Design review of the part built by this model. Coordinates are the model's own, in mm. A direction names the side the tool comes from. Round coordinates to 2 decimals unless told otherwise and drop trailing zeros. Order: outer loops, then holes, each group sorted by start corner. A loop starts at its lowest first (then second) coordinate and runs counter-clockwise, first axis right, second up. Notation, with made-up numbers: (-22, 55) - (-18, 55) arc R21 cw to (-18, 67) - close; hole circle Ø6 at (-34.75, -6.75). An arc over 180 degrees is marked (long way). Answer as a JSON object with one key per item and string values. Group by question number.
from build123d import *

# Parameters (mm, degrees)
F0_R     = 7.625
F0_R_2   = 7
F1_DEPTH = 10.25
F2_DEPTH = 19.75
F3_DEPTH = 28.7
F4_SIZE  = 2.25


with BuildPart() as f1:
    # F0 (on Front) → F1 (new body)
    with BuildSketch(Plane.XZ):
        with BuildLine():
            Line((10.175, 10.075), (-10.075, 10.075))
            Line((-10.075, 10.075), (-10.075, 1.7320508076))
            ThreePointArc((-10.075, 1.7320508076), (-9.3429491924, 1), (-9.075, 0))
            ThreePointArc((-9.075, 0), (-9.3429491924, -1), (-10.075, -1.7320508076))
            Line((-10.075, -1.7320508076), (-10.075, -10.175))
            Line((-10.075, -10.175), (10.175, -10.175))
            Line((10.175, -10.175), (10.175, -1.7820508076))
            ThreePointArc((10.175, -1.7820508076), (9.175, -0.05), (10.175, 1.6820508076))
            Line((10.175, 1.6820508076), (10.175, 10.075))
        make_face()
        Circle(F0_R, mode=Mode.SUBTRACT)
        with BuildLine():
            Line((-10.075, -1.7320508076), (-10.075, 1.7320508076))
            ThreePointArc((-10.075, 1.7320508076), (-13.075, 0), (-10.075, -1.7320508076))
        make_face()
        with BuildLine():
            ThreePointArc((13.175, -0.05), (12.175, 1.6820508076), (10.175, 1.6820508076))
            Line((10.175, 1.6820508076), (10.175, -1.7820508076))
            ThreePointArc((10.175, -1.7820508076), (12.175, -1.7820508076), (13.175, -0.05))
        make_face()
        with BuildLine():
            Line((10.175, -1.7820508076), (10.175, 1.6820508076))
            ThreePointArc((10.175, 1.6820508076), (9.175, -0.05), (10.175, -1.7820508076))
        make_face()
        Circle(F0_R)
        Circle(F0_R_2, mode=Mode.SUBTRACT)
        Circle(F0_R_2)
        with BuildLine():
            ThreePointArc((-9.075, 0), (-9.3429491924, 1), (-10.075, 1.7320508076))
            Line((-10.075, 1.7320508076), (-10.075, -1.7320508076))
            ThreePointArc((-10.075, -1.7320508076), (-9.3429491924, -1), (-9.075, 0))
        make_face()
    extrude(amount=F1_DEPTH)

    # F0 (on Front) → F2 (join)
    with BuildSketch(Plane.XZ):
        Circle(F0_R)
        Circle(F0_R_2, mode=Mode.SUBTRACT)
        Circle(F0_R_2)
    extrude(amount=F2_DEPTH)

    # F0 (on Front) → F3 (join)
    with BuildSketch(Plane.XZ):
        Circle(F0_R_2)
    extrude(amount=F3_DEPTH)

    # F4
    f4_edges = [f1.edges().sort_by_distance(p)[0] for p in [
        (-10.075, -5.125, 10.075),
        (10.175, -5.125, 10.075),
        (10.175, -5.125, -10.175),
        (-10.075, -5.125, -10.175),
    ]]
    chamfer(f4_edges, length=F4_SIZE)


solid = f1.part
1. Take a section at B-B, the plane x = 0. Give the boundary of the cut face in (y, z) (3 decimals), then the cut area to 3 significant figures.
2. Take a section at D-D, the plane y = -18.5. Give the boundary of the cut face in (x, z) (3 decimals).
3. To check wall thickness, follow line 1 (Y direction, x = 7, z = 2.75); line 2 (Y direction, x = 8.25, z = 8.25); line 3 (X direction, y = -5.5, z = -3.25) (3 decimals). State the ranges of each line that lie inside material, in increasing order. Write a range as from..to.
4. Take a section at A-A, the plane y = -2.75. Give the boundary of the cut face in (x, z) (3 decimals).
5. Mouldability with a two-part tool opening along X and no side actions: class faces 3 (the cylindrical face through (-13.074, -5.053, 0.059)), 4 (the cylindrical face through (6.466, -24.162, -2.681)), 5 (the flat face through (-9, -5, -9)), 6 (the flat face through (7, -19.75, -2)) as pulls with the +X half, pulls with the -X half, needs draft (parallel to the pull), parting line crosses it, or undercut.
6. Clearance check with flat-ended pins moving along their axes: P1, Ø3, axis at y = -5.5, z = 4, coming from the -X side (3 decimals); P2, Ø3, axis at y = -4, z = 5, coming from the +X side (3 decimals); P3, Ø6, axis at x = -8.5, z = -6.5, coming from the -Y side. State where each tip first meets the part, or that it passes through.
7. Tool access review of faces 1 (the flat face through (9, -10.25, 0)), 2 (the flat face through (0, 0, 0)): name each direction out of +Z, -Z, +X, -X, +Y, -Y from which nothing blocks a thin tool from reaching the whole face with its end or side.
8. Take a section at C-C, the plane z = -5.75. Give the boundary of the cut face in (x, y) (3 decimals).
Response values:
{
 "1": {"outline": "(-28.7, -7) - (-19.75, -7) - (-19.75, -7.625) - (-10.25, -7.625) - (-10.25, -10.175) - (0, -10.175) - (0, 10.075) - (-10.25, 10.075) - (-10.25, 7.625) - (-19.75, 7.625) - (-19.75, 7) - (-28.7, 7) - close", "area": "478 mm2"},
 "2": {"outline": "circle Ø15.25 at (0, 0)"},
 "3": {"line 1": "-19.75..0", "line 2": "-10.25..0", "line 3": "-10.075..10.175"},
 "4": {"outline": "(-10.075, -7.925) - (-7.825, -10.175) - (7.925, -10.175) - (10.175, -7.925) - (10.175, -1.782) arc R2 ccw (long way) to (10.175, 1.682) - (10.175, 7.825) - (7.925, 10.075) - (-7.825, 10.075) - (-10.075, 7.825) - (-10.075, 1.732) arc R2 ccw (long way) to (-10.075, -1.732) - close"},
 "5": {"face 3": "undercut", "face 4": "parting line crosses it", "face 5": "pulls with the -X half", "face 6": "needs draft"},
 "6": {"P1": "x = -10.075", "P2": "x = 10.175", "P3": "y = -10.25"},
 "7": {"face 1": "-Y", "face 2": "+Z, -Z, +X, -X, +Y"},
 "8": {"outline": "(-10.075, -10.25) - (-5.008, -10.25) - (-5.008, -19.75) - (-3.992, -19.75) - (-3.992, -28.7) - (3.992, -28.7) - (3.992, -19.75) - (5.008, -19.75) - (5.008, -10.25) - (10.175, -10.25) - (10.175, 0) - (-10.075, 0) - close"}
}
